from build123d import *

# Parameters (mm, degrees)
REVOLVE1_ANGLE = 270


with BuildPart() as part:
    # Sketch1 → Revolve1 (revolve)
    with BuildSketch(Plane.XY):
        Polygon((-35, 20), (35, 20), (35, 54), (26.5, 54), (26.5, 108.052540289), (80, 133), (80, 163), (70, 163), (61.539060338, 180), (51.539060338, 180), (42.5, 163), (32.5, 163), (24.039060338, 180), (14.039060338, 180), (5, 163), (-5, 163), (-14.039060338, 180), (-24.039060338, 180), (-32.5, 163), (-42.5, 163), (-51.539060338, 180), (-61.539060338, 180), (-70, 163), (-80, 163), (-80, 133), (-26.5, 108.052540289), (-26.5, 54), (-35, 54), align=None)
    revolve(axis=Axis((0, 0, 0), (-1, 0, 0)), revolution_arc=REVOLVE1_ANGLE)


solid = part.part
Can you work these out from the model? Positions are in its coordinate system, mm. A direction names the side the tool comes from. Give positions to 0.01 mm unless a question says otherwise; leave off trailing zeros. Write each question's results on one line, items separated by ' | '.
1) Please list where these lines run through material, in increasing order: line 1 along X through (y, z) = (-158.5, 56.5); line 2 along X through (y, z) = (-152, 68); line 3 along Y through (x, z) = (69, -48). Write a range as [from, to].
Final values:
line 1: x = [-67.38, -45.3], [-29.88, -7.8], [7.8, 29.88], [45.3, 67.38] | line 2: x = [-68.25, -44.37], [-30.75, -6.87], [6.87, 30.75], [44.37, 68.25] | line 3: y = [-157.87, -118.52], [118.52, 157.87]
2) I'm going to push flat-ended pins straight in: pin 1 Ø10 at (y, z) = (-129.5, 10) entering from -X; pin 2 Ø8 at (y, z) = (52, -77.5) entering from -X; pin 3 Ø2 at (x, y) = (43.5, 83) entering from +Z; pin 4 Ø5 at (x, z) = (34, -69) entering from -Y. Where does each tip first touch, or does it pass through?
Final values:
pin 1: stops at x = -80 | pin 2: stops at x = -26.5 | pin 3: stops at z = -79.77 | pin 4: stops at y = -150.01
3) If we mould it in two halves opening along X, with no side actions, what happens to faces 4 (the face through (18.97, -123.01, -131.41)), 5 (the face through (-26.5, -50, -26)), 6 (the face through (31.971, -112.121, -119.773))? For each: pulls with the +X half, pulls with the -X half, needs draft (parallel to the pull), parting line crosses it, or undercut.
Final values:
face 4: needs draft | face 5: pulls with the -X half | face 6: undercut
4) On a 3-axis mill with a long thin cutter (end or side, diameter ignored), from which of +Z, -Z, +X, -X, +Y, -Y can I reach the whole of each face in a straight line? I mean faces 1 (the face through (35, -23, -13)), 2 (the face through (-1, 0, 119)), 3 (the face through (5.44, -111.96, -119.6)). Say none if no direction works.
Final values:
face 1: +X | face 2: +Z, +X, -X, +Y | face 3: none
